from build123d import *

# Parameters (mm, degrees)
F1_DEPTH = 207
F2_R     = 5
F3_T     = -1


with BuildPart() as f1:
    # F0 (on Top) → F1 (new body)
    with BuildSketch(Plane.XY):
        with BuildLine():
            ThreePointArc((-29.4389327221, -1.8971663562), (-34.2138220516, -4.2365060198), (-35.2552827265, -9.450663462))
            ThreePointArc((-35.2552827265, -9.450663462), (-0.1275131337, -36.4997772651), (35.1883905908, -9.696760677))
            ThreePointArc((35.1883905908, -9.696760677), (34.1833865425, -4.4754538451), (29.4249586801, -2.1028092345))
            Line((29.4249586801, -2.1028092345), (-29.4389327221, -1.8971663562))
        make_face()
    extrude(amount=F1_DEPTH)

    # F2
    f2_edges = [f1.edges().sort_by_distance(p)[0] for p in [
        (-0.127513, -36.499777, 0),
    ]]
    fillet(f2_edges, radius=F2_R)

    # F3
    f3_openings = [f1.faces().sort_by_distance(p)[0] for p in [
        (-0.058469, -16.736236, 207),
    ]]
    offset(amount=F3_T, openings=f3_openings)


solid = f1.part
Can you work these out from the model? Positions are in its coordinate system, mm. A direction names the side the tool comes from. Give positions to 0.01 mm unless a question says otherwise; leave off trailing zeros. Order: outer loops, then holes, each group sorted by start corner. A loop starts at its lowest first (then second) coordinate and runs counter-clockwise, first axis right, second up. Notation, with made-up numbers: (64, 80) - (113, 80) arc R21 cw to (113, 97) - close; hole circle Ø7 at (77, 53). An arc over 180 degrees is marked (long way). Write each question's results on one line, items separated by ' | '.
1) If we mould it in two halves opening along Y, with no side actions, what happens to faces 1 (the face through (-0.2, -2.5, 207)), 2 (the face through (-34.17, -4.18, 104.59)), 3 (the face through (-33.382, -4.796, 104.586))? For each: pulls with the +Y half, pulls with the -Y half, needs draft (parallel to the pull), parting line crosses it, or undercut.
Final values:
face 1: needs draft | face 2: parting line crosses it | face 3: undercut
2) I'm going to push flat-ended pins straight in: pin 1 Ø12 at (x, z) = (-6.5, 27.5) entering from -Y; pin 2 Ø4 at (x, y) = (24.5, -18) entering from +Z; pin 3 Ø5 at (x, y) = (13, -20.5) entering from +Z. Where does each tip first touch, or does it pass through?
Final values:
pin 1: stops at y = -36.5 | pin 2: stops at z = 1.1 | pin 3: stops at z = 1
3) Please list where these lines run through material, in increasing order: line 1 along Z through (x, y) = (9, -12); line 2 along X through (y, z) = (-14.5, 47.5); line 3 along Y through (x, z) = (-18.5, 177.5). Write a range as [from, to].
Final values:
line 1: z = [0, 1] | line 2: x = [-33.5, -32.4], [32.4, 33.5] | line 3: y = [-31.46, -30.3], [-2.94, -1.94]
4) On a 3-axis mill with a long thin cutter (end or side, diameter ignored), from which of +Z, -Z, +X, -X, +Y, -Y can I reach the whole of each face in a straight line? I mean faces 4 (the face through (-0.77, -35.49, 104.59)), 5 (the face through (0, -3, 2)), 6 (the face through (-0.79, -36.49, 104.59)). Say none if no direction works.
Final values:
face 4: +Z | face 5: -Z, +X, +Y | face 6: +Z, -Z, -Y
5) Suppose I cut it at A-A, the plane z = 107. Write out the boundary of the cut face in (x, y), then the cut area to 3 significant figures.
Final values:
outline: (-35.26, -9.45) arc R36.5 ccw to (35.19, -9.7) arc R6 ccw to (29.42, -2.1) - (-29.44, -1.9) arc R6 ccw to start; hole (-34.29, -9.19) arc R35.5 ccw to (34.22, -9.43) arc R5 ccw to (29.42, -3.1) - (-29.44, -2.9) arc R5 ccw to start | area: 173 mm^2
